from build123d import *

# Parameters (mm, degrees)
SKETCH1_R             = 65
BOSS_EXTRUDE1_DEPTH   = 27
SKETCH2_R             = 7.5
CUT_EXTRUDE1_DEPTH    = 96.807097858
SKETCH3_R             = 6.48724829
CUT_EXTRUDE2_DEPTH    = 21.005107
CIRPATTERN1_START     = 5.994892811
CIRPATTERN1_OUTLINE_R = 6.48724829
CIRPATTERN1_DEPTH     = 21.005107189


# Read off the part's stored shape, not the designer's step: CirPattern1
with BuildPart() as part:
    # Sketch1 → Boss-Extrude1 (new body)
    with BuildSketch(Plane(origin=(0, 0, 0), x_dir=(1, 0, 0), z_dir=(0, 1, 0))):
        with Locations(Location((0, 0, 0), (0, 0, 270))):
            Circle(SKETCH1_R)
    extrude(amount=BOSS_EXTRUDE1_DEPTH)

    # Sketch2 → Cut-Extrude1 (cut, through all)
    with BuildSketch(Plane(origin=(0, 0, 0), x_dir=(1, 0, 0), z_dir=(0, 1, 0))):
        with Locations(Location((0, 0, 0), (0, 0, 270))):
            Circle(SKETCH2_R)
    extrude(amount=CUT_EXTRUDE1_DEPTH, mode=Mode.SUBTRACT)

    # Sketch3 → Cut-Extrude2 (cut)
    with BuildSketch(Plane(origin=(0, 27, 0), x_dir=(1, 0, 0), z_dir=(0, 1, 0))):
        with Locations(Location((-16.80132063, 0, 0), (0, 0, 270))):
            Circle(SKETCH3_R)
    extrude(amount=-CUT_EXTRUDE2_DEPTH, mode=Mode.SUBTRACT)

    # CirPattern1 outline → CirPattern1 (cut)
    with BuildSketch(Plane(origin=(0, 0, 0), x_dir=(1, 0, 0), z_dir=(0, 1, 0)).offset(CIRPATTERN1_START)):
        with Locations((-5.191893603, -15.979005467)):
            Circle(CIRPATTERN1_OUTLINE_R)
        with Locations((13.592553918, -9.875568485)):
            Circle(CIRPATTERN1_OUTLINE_R)
        with Locations((13.592553918, 9.875568485)):
            Circle(CIRPATTERN1_OUTLINE_R)
        with Locations((-5.191893603, 15.979005467)):
            Circle(CIRPATTERN1_OUTLINE_R)
    extrude(amount=CIRPATTERN1_DEPTH, mode=Mode.SUBTRACT)


solid = part.part
Geometry: final body of the model. Coordinates: model frame, mm. A direction names the side the tool comes from. Coordinates: 2 decimals unless noted, no trailing zeros. Loops run counter-clockwise (first coordinate to the right, second up) from the corner with the lowest first, then second, coordinate; pieces in that order, holes last. Notation, with made-up numbers: M 15.5,-21 L 39.5,-21 A8 ccw 39.5,-11 Z; hole C -23.75,87 d2. An arc over 180 degrees is marked long. One line per item, written item: value. Start each with the question number.
1) Reachability of faces 1 (the flat face through (15, 27, -1)), 2 (the cylindrical face through (-2.198, 16.35, 21.734)) from +Z, -Z, +X, -X, +Y, -Y: full face, straight path, thin tool, end or side. Return the list, or none.
2) Material intervals for L1, parallel to X at y = 19.5, z = 0; L2, parallel to X at y = 23, z = 13.5; L3, parallel to Z at x = 17, y = 15.25, sorted ascending. Write a range as from..to.
3) Draft query along Y for faces 3 (the cylindrical face through (-22.56, 16.64, 2.99)), 4 (the flat face through (14, 5.995, 10)), 5 (the flat face through (1, 0, 14)). Return one class per face: released by +Y, released by -Y, zero draft, split by the parting line, or undercut.
4) Cut plane D-D (z = 51.5). Return loops of the section in (x, y), then the cut area to 3 significant figures.
5) Cut plane B-B (y = 4). Return loops of the section in (x, z), then the cut area to 3 significant figures.
6) Pin query (flat end, axial travel): P1, Ø6.5, axis at x = -17.5, z = -3, coming from the +Y side; P2, Ø6, axis at x = -18, y = 22.5, coming from the +Z side; P3, Ø1.5, axis at y = 22, z = -40, coming from the -X side. Return the tip coordinate at first contact, or that it passes through.
7) Cut plane A-A (z = 0). Return loops of the section in (x, y), then the cut area to 3 significant figures.
8) Cut plane C-C (y = 25.25). Return loops of the section in (x, z).
Evaluation:
1. face 1: +Z, -Z, +X, -X, +Y
1. face 2: +Y
2. L1: -65..-23.29, -10.31..-7.5, 7.5..65
2. L2: -63.58..-11.19, 0.8..8.21, 18.97..63.58
2. L3: -62.74..-15.4, -4.36..4.36, 15.4..62.74
3. face 3: zero draft
3. face 4: released by +Y
3. face 5: released by -Y
4. outline: M -39.66,0 L 39.66,0 L 39.66,27 L -39.66,27 Z
4. area: 2,140 mm^2
5. outline: C 0,0 d130; hole C 0,0 d15
5. area: 13,100 mm^2
6. P1: y = 5.99
6. P2: z = 63.25
6. P3: x = -51.81
7. outline: M -65,0 L -7.5,0 L -7.5,27 L -10.31,27 L -10.31,5.99 L -23.29,5.99 L -23.29,27 L -65,27 Z; M 7.5,0 L 65,0 L 65,27 L 7.5,27 Z
7. area: 2,830 mm^2
8. outline: C 0,0 d130; hole C -16.8,0 d12.97; hole C -5.19,-15.98 d12.97; hole C -5.19,15.98 d12.97; hole C 0,0 d15; hole C 13.59,-9.88 d12.97; hole C 13.59,9.88 d12.97
